from build123d import *

# Parameters (mm, degrees)
EXTRUDE_THIN1_DEPTH    = 68.2625
SKETCH2_R              = 6.35
CUT_EXTRUDE1_DEPTH     = 266.758121054
FILLET1_R              = 15.875
CUT_EXTRUDE2_DEPTH     = 150.132085435
CONVERT_SOLID1_START   = -68.2625
CONVERT_SOLID1_DEPTH   = 136.525
CONVERT_SOLID1_2_DEPTH = 136.525
SKETCH8_R              = 120.65
CUT_EXTRUDE3_DEPTH     = 150.132085435


# Read off the part's stored shape, not the designer's step: Convert-Solid1
with BuildPart() as part:
    # Sketch1 → Extrude-Thin1 (new, symmetric)
    with BuildSketch(Plane(origin=(0, 0, 0), x_dir=(0, 0, -1), z_dir=(1, 0, 0))):
        Polygon((-127, -38.1), (-127, 0), (127, 0), (127, -38.1), (120.65, -38.1), (120.65, -6.35), (-120.65, -6.35), (-120.65, -38.1), align=None)
    extrude(amount=EXTRUDE_THIN1_DEPTH, both=True)

    # Sketch2 → Cut-Extrude1 (cut, through all)
    with BuildSketch(Plane.XY.offset(127)):
        with Locations((-49.2125, -22.225)):
            Circle(SKETCH2_R)
        with Locations((52.3875, -22.225)):
            Circle(SKETCH2_R)
    extrude(amount=-CUT_EXTRUDE1_DEPTH, mode=Mode.SUBTRACT)

    # Fillet1
    fillet1_edges = [part.edges().sort_by_distance(p)[0] for p in [
        (68.2625, -38.1, -123.825),
        (-68.2625, -38.1, -123.825),
        (68.2625, -38.1, 123.825),
        (-68.2625, -38.1, 123.825),
    ]]
    fillet(fillet1_edges, radius=FILLET1_R)

    # Sketch3 → Cut-Extrude2 (cut, through all)
    with BuildSketch(Plane(origin=(0, 0, 0), x_dir=(1, 0, 0), z_dir=(0, 1, 0))):
        with BuildLine():
            Line((-4.7625, 38.1), (68.2625, 38.1))
            Line((68.2625, 38.1), (68.2625, -38.1))
            Line((68.2625, -38.1), (-4.7625, -38.1))
            ThreePointArc((-4.7625, -38.1), (-42.8625, 0), (-4.7625, 38.1))
        make_face()
    extrude(amount=-CUT_EXTRUDE2_DEPTH, mode=Mode.SUBTRACT)

    # Convert-Solid1 outline → Convert-Solid1 (cut)
    with BuildSketch(Plane.YZ.offset(CONVERT_SOLID1_START)):
        with BuildLine():
            Line((0, -127), (0, -116.84))
            ThreePointArc((0, -116.84), (-2.975795103, -124.024204897), (-10.16, -127))
            Line((-10.16, -127), (0, -127))
        make_face()
        with BuildLine():
            ThreePointArc((-10.16, 127), (-2.975795103, 124.024204897), (0, 116.84))
            Line((0, 116.84), (0, 127))
            Line((0, 127), (-10.16, 127))
        make_face()
    extrude(amount=CONVERT_SOLID1_DEPTH, mode=Mode.SUBTRACT)

    # Convert-Solid1 2 outline → Convert-Solid1 2 (add)
    with BuildSketch(Plane.YZ.offset(CONVERT_SOLID1_START)):
        with BuildLine():
            Line((-6.35, -120.65), (-6.35, -116.84))
            ThreePointArc((-6.35, -116.84), (-7.465923164, -119.534076836), (-10.16, -120.65))
            Line((-10.16, -120.65), (-6.35, -120.65))
        make_face()
        with BuildLine():
            ThreePointArc((-10.16, 120.65), (-7.465923164, 119.534076836), (-6.35, 116.84))
            Line((-6.35, 116.84), (-6.35, 120.65))
            Line((-6.35, 120.65), (-10.16, 120.65))
        make_face()
    extrude(amount=CONVERT_SOLID1_2_DEPTH)

    # Sketch8 → Cut-Extrude3 (cut, through all)
    with BuildSketch(Plane(origin=(0, 0, 0), x_dir=(1, 0, 0), z_dir=(0, 1, 0))):
        with Locations((118.745, 0)):
            Circle(SKETCH8_R)
    extrude(amount=-CUT_EXTRUDE3_DEPTH, mode=Mode.SUBTRACT)


solid = part.part
Here's how the part is built. I have some questions about the finished solid (model axes, mm). A direction names the side the tool comes from. Give positions to 0.01 mm unless a question says otherwise; leave off trailing zeros. Loops run counter-clockwise (first coordinate to the right, second up) from the corner with the lowest first, then second, coordinate; pieces in that order, holes last. Notation, with made-up numbers: (49.5, -13) -> (108.5, -13) arc R25 cw to (108.5, 7) -> close; hole circle Ø7 at (-35.75, 47.25). An arc over 180 degrees is marked (long way). One line per item, written item: value.
Q1. Suppose I cut it at A-A on y = -13. Please give me the cut outline in (x, z).
Answers follow:
outline: (-68.26, -127) -> (68.26, -127) -> (68.26, -120.65) -> (-68.26, -120.65) -> close; (-68.26, 120.65) -> (68.26, 120.65) -> (68.26, 127) -> (-68.26, 127) -> close
Q2. We'd pull the mould along X, two halves only. Please class faces 1 (the face through (63.736, -33.326, -123.781)), 2 (the face through (-55.556, -21.946, -123.781)), 3 (the face through (-0.956, -2.897, -123.945)): pulls with the +X half, pulls with the -X half, needs draft (parallel to the pull), parting line crosses it, or undercut.
Answers follow:
face 1: pulls with the +X half
face 2: undercut
face 3: needs draft
Q3. Suppose I cut it at B-B on x = -48.5. Please give me the cut outline in (y, z).
Answers follow:
outline: (-38.1, -127) -> (-28.53, -127) -> (-28.53, -120.65) -> (-38.1, -120.65) -> close; (-38.1, 120.65) -> (-28.53, 120.65) -> (-28.53, 127) -> (-38.1, 127) -> close; (-15.92, -127) -> (-10.16, -127) arc R10.16 ccw to (0, -116.84) -> (0, 116.84) arc R10.16 ccw to (-10.16, 127) -> (-15.92, 127) -> (-15.92, 120.65) -> (-10.16, 120.65) arc R3.81 cw to (-6.35, 116.84) -> (-6.35, -116.84) arc R3.81 cw to (-10.16, -120.65) -> (-15.92, -120.65) -> close
Q4. Suppose I cut it at C-C on x = 27. Please give me the cut outline in (y, z), then the cut area to 3 significant figures.
Answers follow:
outline: (-38.1, -127) -> (-10.16, -127) arc R10.16 ccw to (0, -116.84) -> (0, -78.35) -> (-6.35, -78.35) -> (-6.35, -116.84) arc R3.81 cw to (-10.16, -120.65) -> (-38.1, -120.65) -> close; (-38.1, 120.65) -> (-10.16, 120.65) arc R3.81 cw to (-6.35, 116.84) -> (-6.35, 78.35) -> (0, 78.35) -> (0, 116.84) arc R10.16 ccw to (-10.16, 127) -> (-38.1, 127) -> close
area: 983 mm^2
Q5. Suppose I cut it at D-D on y = -26. Please give me the cut outline in (x, z), then the cut area to 3 significant figures.
Answers follow:
outline: (-67.81, -127) -> (-54.32, -127) -> (-54.32, -120.65) -> (-67.81, -120.65) -> close; (-67.81, 120.65) -> (-54.32, 120.65) -> (-54.32, 127) -> (-67.81, 127) -> close; (-44.11, -127) -> (47.28, -127) -> (47.28, -120.65) -> (-44.11, -120.65) -> close; (-44.11, 120.65) -> (47.28, 120.65) -> (47.28, 127) -> (-44.11, 127) -> close; (57.49, -127) -> (67.81, -127) -> (67.81, -120.65) -> (57.49, -120.65) -> close; (57.49, 120.65) -> (67.81, 120.65) -> (67.81, 127) -> (57.49, 127) -> close
area: 1,460 mm^2
Q6. If I drill on line 1 along Z through (x, y) = (-2.5, -35); line 2 along Y through (x, z) = (1, -83), over which ranges is the centre line in solid material (lowest first)?
Answers follow:
line 1: -127 to -120.65, 120.65 to 127
line 2: -6.35 to 0
Q7. On a 3-axis mill with a long thin cutter (end or side, diameter ignored), from which of +Z, -Z, +X, -X, +Y, -Y can I reach the whole of each face in a straight line? I mean faces 4 (the face through (-63.49, -33.57, 123.87)), 5 (the face through (29.32, -3.13, -80.99)), 6 (the face through (1, -24, -120.65)). Say none if no direction works.
Answers follow:
face 4: +Z, -Z, -X, -Y
face 5: +X, +Y, -Y
face 6: +X, -X, -Y
Q8. I'm going to push flat-ended pins straight in: pin 1 Ø7 at (x, y) = (0.5, -4) entering from +Z; pin 2 Ø1 at (y, z) = (-6.5, 84.5) entering from -X; pin 3 Ø1.5 at (x, y) = (16.5, -5) entering from -Z; pin 4 Ø5 at (x, y) = (2, -4.5) entering from -Z. Where does each tip first touch, or does it pass through?
Answers follow:
pin 1: z = 126.65
pin 2: x = -68.26
pin 3: z = -125.99
pin 4: z = -126.5
